Could you check a few things on this model? Use its own coordinates, in mm. A direction names the side the tool comes from. Coordinates: 2 decimals unless noted, no trailing zeros. Order: outer loops, then holes, each group sorted by start corner. A loop starts at its lowest first (then second) coordinate and runs counter-clockwise, first axis right, second up. Notation, with made-up numbers: M -25,-23.5 L 34,-23.5 A22 ccw 34,-1.5 Z; hole C 78,-27.5 d10. An arc over 180 degrees is marked long. Write item = value, one per line. Start each with the question number.
from build123d import *

# Parameters (mm, degrees)
SALIENTE_EXTRUIR1_DEPTH = 200


with BuildPart() as part:
    # Croquis1 → Saliente-Extruir1 (new body)
    with BuildSketch(Plane(origin=(0, 0, 0), x_dir=(0, 0, -1), z_dir=(1, 0, 0))):
        with BuildLine():
            Line((0, 0), (-22.597979746, 0))
            ThreePointArc((-22.597979746, 0), (-23.363346611, 0.152240935), (-24.012193309, 0.585786438))
            Line((-24.012193309, 0.585786438), (-37.656854249, 14.230447378))
            ThreePointArc((-37.656854249, 14.230447378), (-39.39103626, 22.948769087), (-32, 27.887301628))
            Line((-32, 27.887301628), (-24, 27.887301628))
            ThreePointArc((-24, 27.887301628), (-22.585786438, 28.473088065), (-22, 29.887301628))
            Line((-22, 29.887301628), (-22, 42.887301628))
            ThreePointArc((-22, 42.887301628), (-22.152240935, 43.652668493), (-22.585786438, 44.30151519))
            Line((-22.585786438, 44.30151519), (-39.121320344, 60.837049096))
            ThreePointArc((-39.121320344, 60.837049096), (-39.771638598, 64.106419737), (-37, 65.95836944))
            Line((-37, 65.95836944), (-32, 65.95836944))
            ThreePointArc((-32, 65.95836944), (-30.585786438, 66.544155877), (-30, 67.95836944))
            Line((-30, 67.95836944), (-30, 77.95836944))
            ThreePointArc((-30, 77.95836944), (-30.152240935, 78.723736304), (-30.585786438, 79.372583002))
            Line((-30.585786438, 79.372583002), (-35.606601718, 84.393398282))
            ThreePointArc((-35.606601718, 84.393398282), (-38.858192988, 100.740251485), (-25, 110))
            Line((-25, 110), (0, 110))
            Line((0, 110), (0, 0))
        make_face()
    extrude(amount=SALIENTE_EXTRUIR1_DEPTH)


solid = part.part
(1) Please list where these lines run through material, in increasing order: probe 1 along Y at (x, z) = (124.5, 38); probe 2 along Z at (x, y) = (126.5, 19.5); probe 3 along Y at (x, z) = (83, 22.5). Write a range as from..to.
(2) Will these pins go through, and if not, where does the flat tip stop? P1, Ø5, axis at x = 93.5, y = 73.5, coming from the +Z side; P2, Ø6.5, axis at x = 70.5, y = 38.5, coming from the +Z side; P3, Ø1.5, axis at x = 88, z = 33.5, coming from the +Y side.
(3) Imagine slicing it at B-B on y = 23. List the corners of the cut face in (x, z) for me, plus the area to 3 significant figures.
(4) Imagine slicing it at A-A on x = 148. List the corners of the cut face in (y, z) for me, plus the area to 3 significant figures.
(5) Imagine slicing it at C-C on y = 73. List the corners of the cut face in (x, z) for me, plus the area to 3 significant figures.
(6) For faces 1 (the flat face through (99, 110, 13)), 2 (the flat face through (98.6, 81.848, 33.061)), which set-ups out of +Z, -Z, +X, -X, +Y, -Y let a thin tool reach every point of the face, with its end or its side?
Response:
q1.probe_1 = 14.6..25.18, 59.72..65.79, 87.52..102.48
q1.probe_2 = 0..39.99
q1.probe_3 = 0..28.56, 44.21..110
q2.P1 = 30
q2.P2 = 22
q2.P3 = 107.84
q3.outline = M 0,0 L 200,0 L 200,39.37 L 0,39.37 Z
q3.area = 7,870 mm2
q4.outline = M 0,0 L 110,0 L 110,25 A15 ccw 84.39,35.61 L 79.37,30.59 A2 cw 77.96,30 L 67.96,30 A2 cw 65.96,32 L 65.96,37 A3 ccw 60.84,39.12 L 44.3,22.59 A2 cw 42.89,22 L 29.89,22 A2 cw 27.89,24 L 27.89,32 A8 ccw 14.23,37.66 L 0.59,24.01 A2 ccw 0,22.6 Z
q4.area = 3,570 mm2
q5.outline = M 0,0 L 200,0 L 200,30 L 0,30 Z
q5.area = 6,000 mm2
q6.face_1 = +Z, -Z, +X, -X, +Y
q6.face_2 = +Z, +X, -X
